The drawing under review shows one solid part. Ordinate dimensions are in mm from its lowest x, y, z. A direction names the side the tool comes from. Coordinates: 2 decimals unless noted, no trailing zeros. Order: outer loops, then holes, each group sorted by start corner. A loop starts at its lowest first (then second) coordinate and runs counter-clockwise, first axis right, second up.
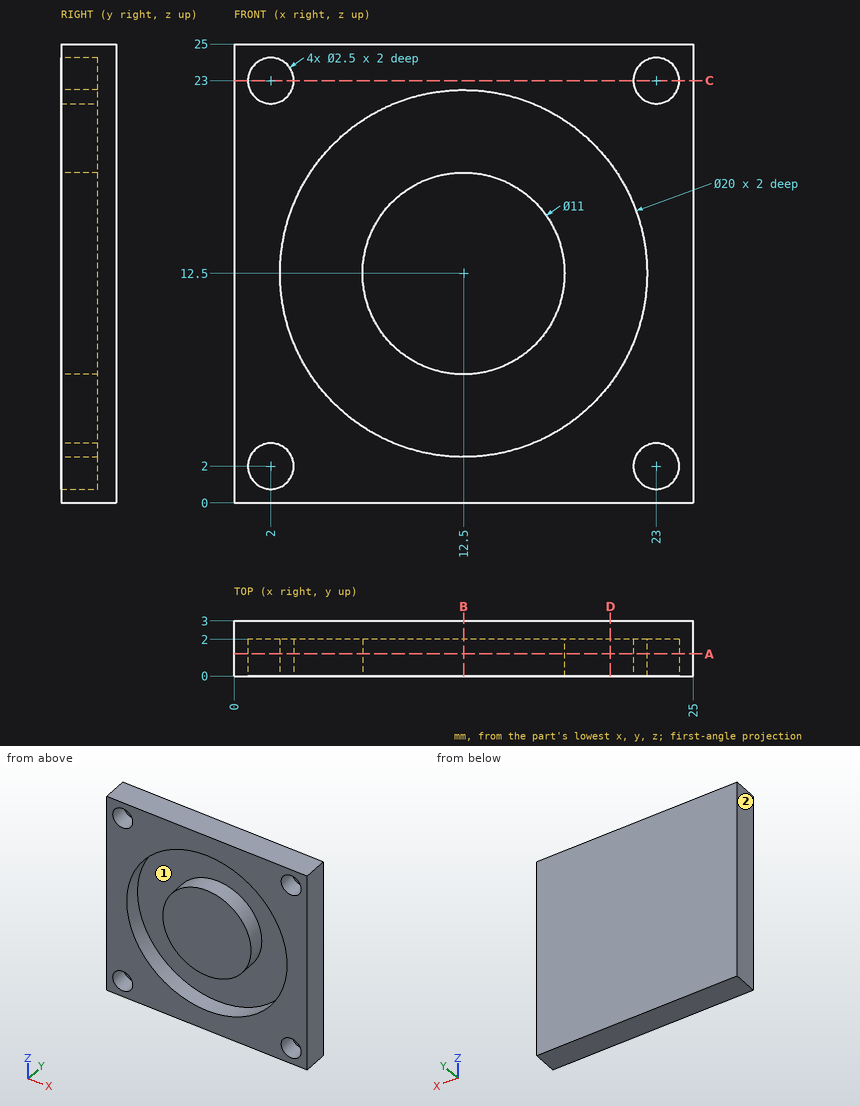
(1) Machinability: for the marked faces 1 and 2, which of the approach directions +Z, -Z, +X, -X, +Y, -Y give a long, thin tool a straight path to every point of the face, cutting with its end or side? Answer none if there is none.
A:
face 1: -Y
face 2: +Z, -Z, -X, +Y, -Y
(2) We need section B-B, the plane x = 12.5. Write out the cut boundary in (y, z), and give its area (3 significant figures).
A:
outline: (0, 0) - (3, 0) - (3, 25) - (0, 25) - (0, 22.5) - (2, 22.5) - (2, 18) - (0, 18) - (0, 7) - (2, 7) - (2, 2.5) - (0, 2.5) - close
area: 57.0 mm2
(3) For pin 1 Ø2 at (x, z) = (23, 2) entering from -Y, flat-tipped, find the tip position at first contact; note if it passes through.
A:
pin 1: stops at y = 2
(4) We need section C-C, the plane z = 23. Write out the cut boundary in (x, y), and give its area (3 significant figures).
A:
outline: (0, 0) - (0.75, 0) - (0.75, 2) - (3.25, 2) - (3.25, 0) - (21.75, 0) - (21.75, 2) - (24.25, 2) - (24.25, 0) - (25, 0) - (25, 3) - (0, 3) - close
area: 65.0 mm2
(5) We need section D-D, the plane x = 20.5. Write out the cut boundary in (y, z), and give its area (3 significant figures).
A:
outline: (0, 0) - (3, 0) - (3, 25) - (0, 25) - (0, 18.5) - (2, 18.5) - (2, 6.5) - (0, 6.5) - close
area: 51.0 mm2
(6) We need section A-A, the plane y = 1.2. Write out the cut boundary in (x, z).
A:
outline: (0, 0) - (25, 0) - (25, 25) - (0, 25) - close; circle Ø11 at (12.5, 12.5); hole circle Ø2.5 at (2, 2); hole circle Ø2.5 at (2, 23); hole circle Ø20 at (12.5, 12.5); hole circle Ø2.5 at (23, 2); hole circle Ø2.5 at (23, 23)
(7) Wall thickness on probe 1 along X at (y, z) = (1.2, 23); probe 2 along X at (y, z) = (1.2, 12.5); probe 3 along Z at (x, y) = (22.75, 1.65): over which ranges is each line inside the solid? List them lowest first.
A:
probe 1: x = 0 to 0.75, 3.25 to 21.75, 24.25 to 25
probe 2: x = 0 to 2.5, 7 to 18, 22.5 to 25
probe 3: z = 0 to 0.78, 3.22 to 21.78, 24.22 to 25
